Read the model definition and answer for the solid it produces. Units are mm, in the model's axes. Face numbers are marked on the shaded views. A direction names the side the tool comes from. Coordinates: 2 decimals unless noted, no trailing zeros. Loops run counter-clockwise (first coordinate to the right, second up) from the corner with the lowest first, then second, coordinate; pieces in that order, holes last.
from build123d import *

# Parameters (mm, degrees)
F1_DEPTH = 3
F2_R     = 1
F3_DEPTH = 3


with BuildPart() as f1:
    # F0 (on Top) → F1 (new body)
    with BuildSketch(Plane.XY):
        with BuildLine():
            ThreePointArc((4.999764, -0.048624), (4.999941, -0.024312), (5, 0))
            ThreePointArc((5, 0), (4.999941, 0.024312), (4.999764, 0.048624))
            ThreePointArc((4.999764, 0.048624), (4.755283, 1.545085), (4.073474, 2.89945))
            ThreePointArc((4.073474, 2.89945), (4.045085, 2.938926), (4.016313, 2.978125))
            ThreePointArc((4.016313, 2.978125), (2.938926, 4.045085), (1.591256, 4.740032))
            ThreePointArc((1.591256, 4.740032), (1.545085, 4.755283), (1.498768, 4.770083))
            ThreePointArc((1.498768, 4.770083), (0, 5), (-1.498768, 4.770083))
            ThreePointArc((-1.498768, 4.770083), (-1.545085, 4.755283), (-1.591256, 4.740032))
            ThreePointArc((-1.591256, 4.740032), (-2.938926, 4.045085), (-4.016313, 2.978125))
            ThreePointArc((-4.016313, 2.978125), (-4.045085, 2.938926), (-4.073474, 2.89945))
            ThreePointArc((-4.073474, 2.89945), (-4.755283, 1.545085), (-4.999764, 0.048624))
            ThreePointArc((-4.999764, 0.048624), (-5, 0), (-4.999764, -0.048624))
            ThreePointArc((-4.999764, -0.048624), (-4.755283, -1.545085), (-4.073474, -2.89945))
            ThreePointArc((-4.073474, -2.89945), (-4.045085, -2.938926), (-4.016313, -2.978125))
            ThreePointArc((-4.016313, -2.978125), (-2.938926, -4.045085), (-1.591256, -4.740032))
            ThreePointArc((-1.591256, -4.740032), (-1.545085, -4.755283), (-1.498768, -4.770083))
            ThreePointArc((-1.498768, -4.770083), (0, -5), (1.498768, -4.770083))
            ThreePointArc((1.498768, -4.770083), (1.545085, -4.755283), (1.591256, -4.740032))
            ThreePointArc((1.591256, -4.740032), (2.938926, -4.045085), (4.016313, -2.978125))
            ThreePointArc((4.016313, -2.978125), (4.045085, -2.938926), (4.073474, -2.89945))
            ThreePointArc((4.073474, -2.89945), (4.755283, -1.545085), (4.999764, -0.048624))
        make_face()
        with BuildLine():
            ThreePointArc((4.073474, 2.89945), (4.755283, 1.545085), (4.999764, 0.048624))
            Line((4.999764, 0.048624), (6.336376, 1.533082))
            Line((6.336376, 1.533082), (6.181867, 2.00861))
            Line((6.181867, 2.00861), (6.027359, 2.484139))
            Line((6.027359, 2.484139), (4.073474, 2.89945))
        make_face()
        with BuildLine():
            Line((6.336376, -1.533082), (4.999764, -0.048624))
            ThreePointArc((4.999764, -0.048624), (4.755283, -1.545085), (4.073474, -2.89945))
            Line((4.073474, -2.89945), (6.027359, -2.484139))
            Line((6.027359, -2.484139), (6.181867, -2.00861))
            Line((6.181867, -2.00861), (6.336376, -1.533082))
        make_face()
        with BuildLine():
            ThreePointArc((1.591256, 4.740032), (2.938926, 4.045085), (4.016313, 2.978125))
            Line((4.016313, 2.978125), (4.225113, 4.964718))
            Line((4.225113, 4.964718), (3.820604, 5.25861))
            Line((3.820604, 5.25861), (3.416096, 5.552503))
            Line((3.416096, 5.552503), (1.591256, 4.740032))
        make_face()
        with BuildLine():
            Line((4.225113, -4.964718), (4.016313, -2.978125))
            ThreePointArc((4.016313, -2.978125), (2.938926, -4.045085), (1.591256, -4.740032))
            Line((1.591256, -4.740032), (3.416096, -5.552503))
            Line((3.416096, -5.552503), (3.820604, -5.25861))
            Line((3.820604, -5.25861), (4.225113, -4.964718))
        make_face()
        with BuildLine():
            ThreePointArc((-1.498768, 4.770083), (0, 5), (1.498768, 4.770083))
            Line((1.498768, 4.770083), (0.5, 6.5))
            Line((0.5, 6.5), (0, 6.5))
            Line((0, 6.5), (-0.5, 6.5))
            Line((-0.5, 6.5), (-1.498768, 4.770083))
        make_face()
        with BuildLine():
            Line((0.5, -6.5), (1.498768, -4.770083))
            ThreePointArc((1.498768, -4.770083), (0, -5), (-1.498768, -4.770083))
            Line((-1.498768, -4.770083), (-0.5, -6.5))
            Line((-0.5, -6.5), (0, -6.5))
            Line((0, -6.5), (0.5, -6.5))
        make_face()
        with BuildLine():
            ThreePointArc((-4.016313, 2.978125), (-2.938926, 4.045085), (-1.591256, 4.740032))
            Line((-1.591256, 4.740032), (-3.416096, 5.552503))
            Line((-3.416096, 5.552503), (-3.820604, 5.25861))
            Line((-3.820604, 5.25861), (-4.225113, 4.964718))
            Line((-4.225113, 4.964718), (-4.016313, 2.978125))
        make_face()
        with BuildLine():
            Line((-3.416096, -5.552503), (-1.591256, -4.740032))
            ThreePointArc((-1.591256, -4.740032), (-2.938926, -4.045085), (-4.016313, -2.978125))
            Line((-4.016313, -2.978125), (-4.225113, -4.964718))
            Line((-4.225113, -4.964718), (-3.820604, -5.25861))
            Line((-3.820604, -5.25861), (-3.416096, -5.552503))
        make_face()
        with BuildLine():
            ThreePointArc((-4.999764, 0.048624), (-4.755283, 1.545085), (-4.073474, 2.89945))
            Line((-4.073474, 2.89945), (-6.027359, 2.484139))
            Line((-6.027359, 2.484139), (-6.181867, 2.00861))
            Line((-6.181867, 2.00861), (-6.336376, 1.533082))
            Line((-6.336376, 1.533082), (-4.999764, 0.048624))
        make_face()
        with BuildLine():
            Line((-6.027359, -2.484139), (-4.073474, -2.89945))
            ThreePointArc((-4.073474, -2.89945), (-4.755283, -1.545085), (-4.999764, -0.048624))
            Line((-4.999764, -0.048624), (-6.336376, -1.533082))
            Line((-6.336376, -1.533082), (-6.181867, -2.00861))
            Line((-6.181867, -2.00861), (-6.027359, -2.484139))
        make_face()
    extrude(amount=F1_DEPTH)

    # F2 (on face) → F3 (cut, through all)
    with BuildSketch(Plane.XY.offset(3)):
        Circle(F2_R)
    extrude(amount=-F3_DEPTH, mode=Mode.SUBTRACT)


solid = f1.part
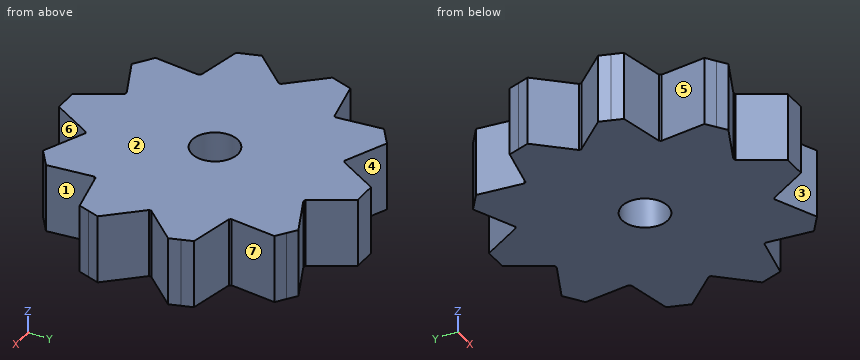
Item 1: A cutting plane is placed at C-C on x = 4.5. Determine the outline of the cut face in (y, z).
Numbers:
outline: (-2.81, 0) - (2.81, 0) - (2.81, 3) - (-2.81, 3) - close
Item 2: A cutting plane is placed at A-A on x = 0. Determine the outline of the cut face in (y, z).
Numbers:
outline: (-6.5, 0) - (-1, 0) - (-1, 3) - (-6.5, 3) - close; (1, 0) - (6.5, 0) - (6.5, 3) - (1, 3) - close
Item 3: Given pin 1 (1.8 mm diameter, centred on x = 0, y = 0, fed in from -Z); pin 2 (1 mm diameter, centred on x = 4.5, z = 2, fed in from -Y), each flat-ended and moving along its own axis, determine where each tip first touches the part or whether it passes through.
Numbers:
pin 1: passes through
pin 2: stops at y = -5.13
Item 4: A cutting plane is placed at B-B on y = 5.75. Determine the outline of the cut face in (x, z).
Numbers:
outline: (-0.93, 0) - (0.93, 0) - (0.93, 3) - (-0.93, 3) - close
Item 5: Determine the mould class of the marked faces 1, 2, 3 and 4 for opening direction X: released by +X, released by -X, zero draft, split by the parting line, or undercut.
Numbers:
face 1: released by +X
face 2: zero draft
face 3: undercut
face 4: undercut
Item 6: Which of the six approach directions +Z, -Z, +X, -X, +Y, -Y give full straight-line access (tool end or side, diameter ignored) to the marked faces 5, 6 and 7?
Numbers:
face 5: +Z, -Z, -X
face 6: +Z, -Z, -Y
face 7: +Z, -Z, +X
Item 7: Find the intervals of material crossed by line 1 along Y through (x, z) = (0, 1.8); line 2 along X through (y, z) = (5.25, 0.25); line 3 along X through (y, z) = (5, 2.3), in increasing order.
Numbers:
line 1: y = -6.5 to -1, 1 to 6.5
line 2: x = -3.83 to -2.74, -1.22 to 1.22, 2.74 to 3.83
line 3: x = -4.18 to -2.18, -1.37 to 1.37, 2.18 to 4.18
